Input: dimensioned drawing with shaded views. Units: mm. Origin: part minimum x, y, z. A direction names the side the tool comes from. Give positions to 0.01 mm unless a question says otherwise; leave off trailing zeros. Order: outer loops, then holes, each group sorted by start corner. A loop starts at its lowest first (then second) coordinate and runs counter-clockwise, first axis right, second up.
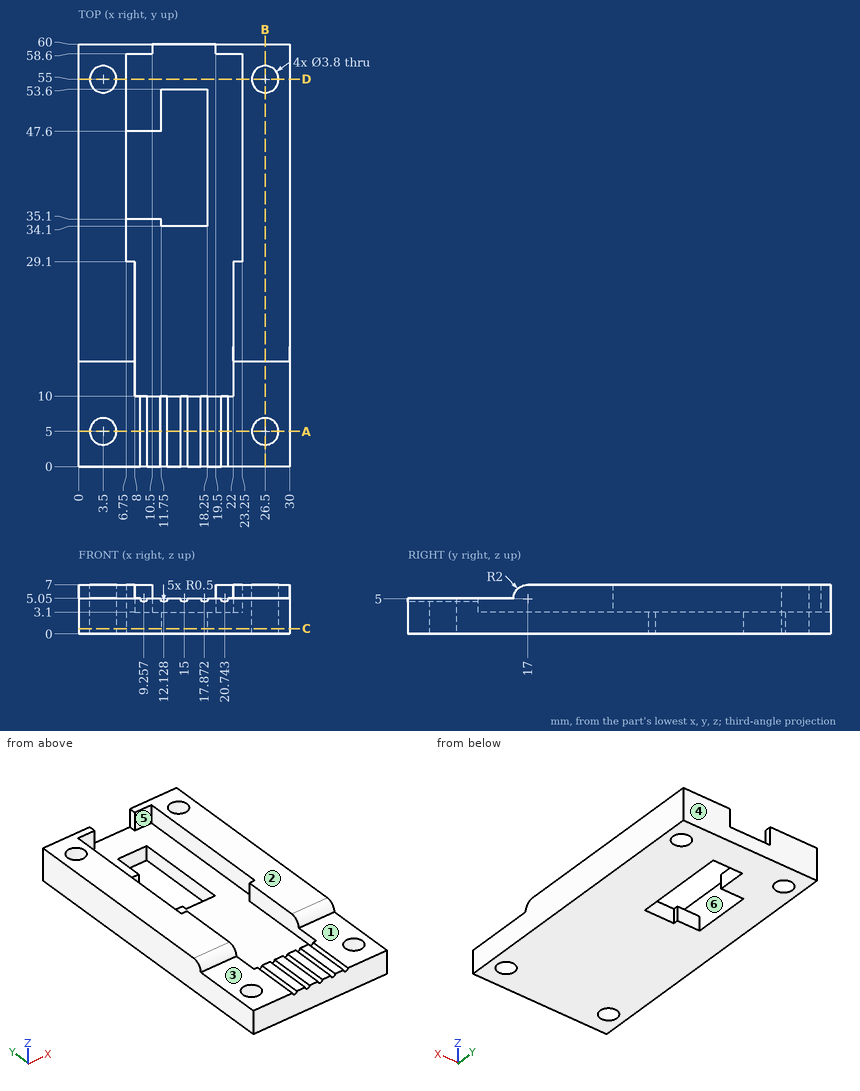
1) Material intervals for L1, parallel to Y at x = 26.5, z = 5; L2, parallel to X at y = 55, z = 5.5; L3, parallel to X at y = 55, z = 1.5, sorted ascending.
Report:
L1: y = 0 to 3.1, 6.9 to 53.1, 56.9 to 60
L2: x = 0 to 1.6, 5.4 to 6.75, 23.25 to 24.6, 28.4 to 30
L3: x = 0 to 1.6, 5.4 to 24.6, 28.4 to 30
2) Reachability of the marked faces 1 and 2 from +Z, -Z, +X, -X, +Y, -Y: full face, straight path, thin tool, end or side. Return the list, or none.
Report:
face 1: +Z, +X, -X, -Y
face 2: +Z, +X, -X, +Y, -Y
3) Section query B-B, the plane x = 26.5. Return the cut outline in (y, z).
Report:
outline: (0, 0) - (3.1, 0) - (3.1, 5.05) - (0, 5.05) - close; (6.9, 0) - (53.1, 0) - (53.1, 7) - (17, 7) arc R2 ccw to (15, 5.05) - (6.9, 5.05) - close; (56.9, 0) - (60, 0) - (60, 7) - (56.9, 7) - close
4) Section query C-C, the plane z = 0.75. Return the cut outline in (x, y), and give its area (3 significant figures).
Report:
outline: (0, 0) - (30, 0) - (30, 60) - (0, 60) - close; hole circle Ø3.8 at (3.5, 5); hole circle Ø3.8 at (3.5, 55); hole (6.75, 35.1) - (11.75, 35.1) - (11.75, 34.1) - (18.25, 34.1) - (18.25, 53.6) - (11.75, 53.6) - (11.75, 47.6) - (6.75, 47.6) - close; hole circle Ø3.8 at (26.5, 5); hole circle Ø3.8 at (26.5, 55)
area: 1,570 mm2
5) Pin query (flat end, axial travel): pin 1 (6 mm diameter, centred on x = 3.5, y = 5, fed in from +Z). Return the tip coordinate at first contact, or that it passes through.
Report:
pin 1: stops at z = 5.05
6) Section query D-D, the plane y = 55. Return the cut outline in (x, z).
Report:
outline: (0, 0) - (1.6, 0) - (1.6, 7) - (0, 7) - close; (5.4, 0) - (24.6, 0) - (24.6, 7) - (23.25, 7) - (23.25, 3.1) - (6.75, 3.1) - (6.75, 7) - (5.4, 7) - close; (28.4, 0) - (30, 0) - (30, 7) - (28.4, 7) - close
7) Section query A-A, the plane y = 5. Return the cut outline in (x, z), and give its area (3 significant figures).
Report:
outline: (0, 0) - (1.6, 0) - (1.6, 5.05) - (0, 5.05) - close; (5.4, 0) - (24.6, 0) - (24.6, 5.05) - (21.24, 5.05) arc R0.5 cw to (20.24, 5.05) - (18.37, 5.05) arc R0.5 cw to (17.37, 5.05) - (15.5, 5.05) arc R0.5 cw to (14.5, 5.05) - (12.63, 5.05) arc R0.5 cw to (11.63, 5.05) - (9.76, 5.05) arc R0.5 cw to (8.76, 5.05) - (5.4, 5.05) - close; (28.4, 0) - (30, 0) - (30, 5.05) - (28.4, 5.05) - close
area: 111 mm2
8) Draft query along Y for the marked faces 3, 4, 5 and 6. Return one class per face: +Y half, -Y half, draft (parallel to the pull), parting line (faces both ways), or undercut.
Report:
face 3: draft
face 4: +Y half
face 5: undercut
face 6: undercut
